Geometry: final body of the model. Coordinates: model frame, mm. A direction names the side the tool comes from. Round coordinates to 2 decimals unless told otherwise and drop trailing zeros. Loops run counter-clockwise (first coordinate to the right, second up) from the corner with the lowest first, then second, coordinate; pieces in that order, holes last. Notation, with made-up numbers: (4.5, 51.25) - (42.5, 51.25) arc R16 cw to (42.5, 71.25) - close; hole circle Ø2 at (26.5, 57). An arc over 180 degrees is marked (long way). Write item = value, one per line. Start each with the question number.
Item 1: Line query: line 1 (Y direction, x = 13.5, z = -23.5) (3 decimals); line 2 (Z direction, x = 8, y = 14.5) (3 decimals); line 3 (X direction, y = -1, z = -22.5). Output: solid intervals per line, ascending. Write a range as from..to.
Item 2: Section B-B (z = -10.75). Return loops of the section in (x, y) (3 decimals), plus the area to 3 significant figures.
Item 3: First-contact query: pin 1 (5 mm diameter, centred on y = -12, z = -12, fed in from +X) (3 decimals); pin 2 (6 mm diameter, centred on x = 14, y = -12.5, fed in from +Z) (3 decimals). Flat tips, straight axial feed; report the tip coordinate or a pass-through.
Item 4: Access query for faces 4 (the flat face through (3.175, -4, -10)), 5 (the cylindrical face through (1.565, 0.07, -15.874)), 6 (the flat face through (16, 3.175, -24)). Directions: +Z, -Z, +X, -X, +Y, -Y. A direction counts if a zero-diameter tool reaches every point of the face in a straight line with its end or side. Return the directions, or none.
Item 5: Draft query along X for faces 1 (the flat face through (2, 0, 0)), 2 (the cylindrical face through (22.224, 0.07, -23.79)), 3 (the cylindrical face through (4.08, -0.22, -21.27)). Return one class per face: pulls with the +X half, pulls with the -X half, needs draft (parallel to the pull), parting line crosses it, or undercut.
Item 6: Section D-D (y = -12). Return loops of the section in (x, z) (3 decimals), plus the area to 3 significant figures.
Item 7: Section C-C (x = 15.75). Return loops of the section in (y, z) (3 decimals).
Item 8: Section A-A (y = 0). Return loops of the section in (x, z) (3 decimals), plus the area to 3 significant figures.
from build123d import *

# Parameters (mm, degrees)
SKETCH3_W          = 3.175
SKETCH3_H          = 31.75
FILLET1_R          = 3.175
FILLET2_R          = 6.35
CUT_EXTRUDE2_REACH = 41.273
CUT_EXTRUDE3_DEPTH = 38.297804895


with BuildPart() as part:
    # Sweep1: sweep along a path in Sketch4
    with BuildLine(Plane(origin=(0, 0, 0), x_dir=(1, 0, 0), z_dir=(0, 1, 0))) as sweep1_path:
        Line((0, 0), (0, 25.4))
        Line((0, 25.4), (25.4, 25.4))
    # Sketch3 → Sweep1 (sweep)
    with BuildSketch(Plane.XY):
        with Locations((1.5875, 0)):
            Rectangle(SKETCH3_W, SKETCH3_H)
    sweep(path=sweep1_path.line, transition=Transition.RIGHT)

    # Fillet1
    fillet1_edges = [part.edges().sort_by_distance(p)[0] for p in [
        (3.175, 0, -22.225),
    ]]
    fillet(fillet1_edges, radius=FILLET1_R)

    # Fillet2
    fillet2_edges = [part.edges().sort_by_distance(p)[0] for p in [
        (0, 0, -25.4),
    ]]
    fillet(fillet2_edges, radius=FILLET2_R)

    # Sketch6 → Cut-Extrude2 (cut, up to next)
    with BuildSketch(Plane(origin=(0, 0, 0), x_dir=(0, 0, -1), z_dir=(1, 0, 0)), mode=Mode.PRIVATE) as cut_extrude2_sk1:
        with BuildLine():
            Line((12.7, -3.175), (6.35, -3.175))
            ThreePointArc((6.35, -3.175), (3.175, 0), (6.35, 3.175))
            Line((6.35, 3.175), (12.7, 3.175))
            ThreePointArc((12.7, 3.175), (15.875, 0), (12.7, -3.175))
        make_face()
    cut_extrude2_tool1 = extrude(cut_extrude2_sk1.sketch, amount=CUT_EXTRUDE2_REACH, mode=Mode.PRIVATE) & part.part
    add(cut_extrude2_tool1.solids().sort_by_distance((0, 0, -9.525))[0], mode=Mode.SUBTRACT)

    # Sketch7 → Cut-Extrude3 (cut, through all)
    with BuildSketch(Plane.XY.offset(-22.225)):
        with BuildLine():
            Line((12.7, 3.175), (19.05, 3.175))
            ThreePointArc((19.05, 3.175), (22.225, 0), (19.05, -3.175))
            Line((19.05, -3.175), (12.7, -3.175))
            ThreePointArc((12.7, -3.175), (9.525, 0), (12.7, 3.175))
        make_face()
    extrude(amount=-CUT_EXTRUDE3_DEPTH, mode=Mode.SUBTRACT)


solid = part.part
Taken from the geometry:
q1.line_1 = -15.875..-3.175, 3.175..15.875
q1.line_2 = -25.4..-22.225
q1.line_3 = 1.02..9.69, 22.06..25.4
q2.outline = (0, -15.875) - (3.175, -15.875) - (3.175, -3.175) - (0, -3.175) - close; (0, 3.175) - (3.175, 3.175) - (3.175, 15.875) - (0, 15.875) - close
q2.area = 80.6 mm^2
q3.pin_1 = 3.175
q3.pin_2 = -22.225
q4.face_4 = +Z, +X, +Y, -Y
q4.face_5 = +X, -X
q4.face_6 = +Z, -Z
q5.face_1 = needs draft
q5.face_2 = undercut
q5.face_3 = pulls with the +X half
q6.outline = (0, -19.05) arc R6.35 ccw to (6.35, -25.4) - (25.4, -25.4) - (25.4, -22.225) - (6.35, -22.225) arc R3.175 cw to (3.175, -19.05) - (3.175, 0) - (0, 0) - close
q6.area = 145 mm^2
q7.outline = (-15.875, -25.4) - (-3.175, -25.4) - (-3.175, -22.225) - (-15.875, -22.225) - close; (3.175, -25.4) - (15.875, -25.4) - (15.875, -22.225) - (3.175, -22.225) - close
q8.outline = (0, -19.05) arc R6.35 ccw to (6.35, -25.4) - (9.525, -25.4) - (9.525, -22.225) - (6.35, -22.225) arc R3.175 cw to (3.175, -19.05) - (3.175, -15.875) - (0, -15.875) - close; (0, -3.175) - (3.175, -3.175) - (3.175, 0) - (0, 0) - close; (22.225, -25.4) - (25.4, -25.4) - (25.4, -22.225) - (22.225, -22.225) - close
q8.area = 64.1 mm^2
